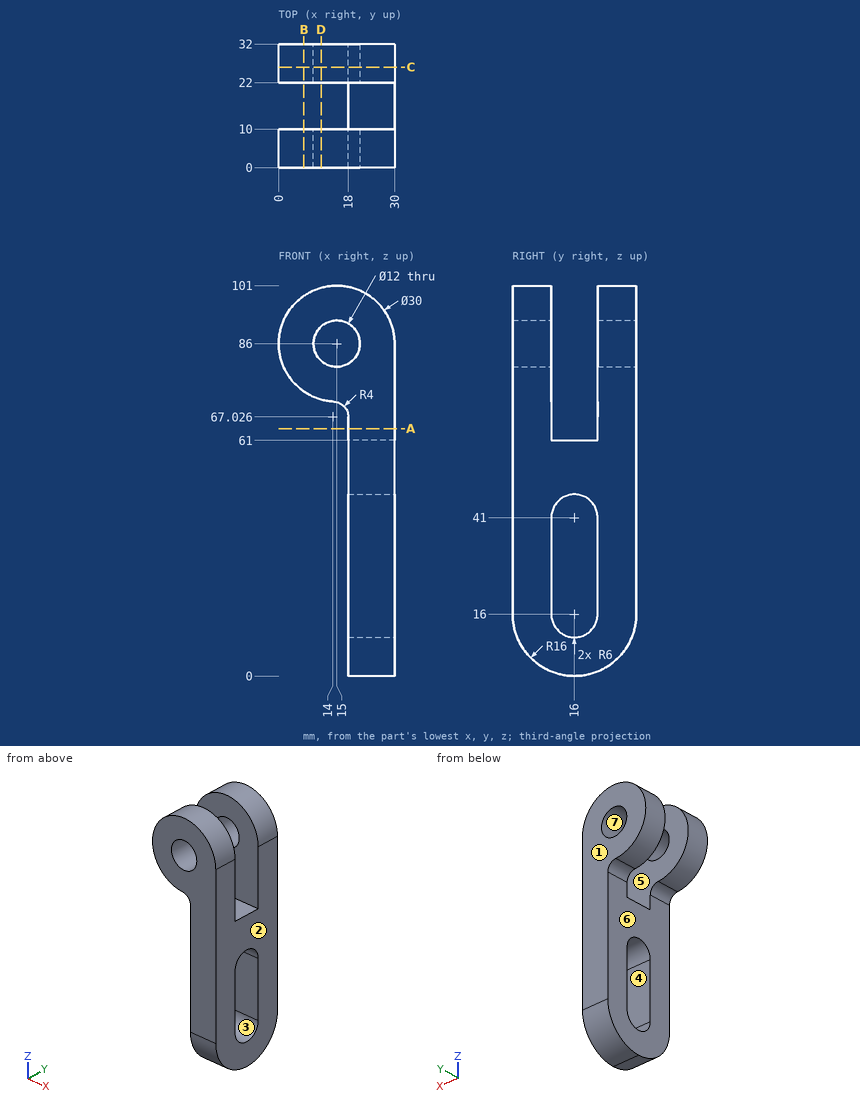
For this review, use the dimensioned drawing (mm, ordinates from the lowest corner) and the shaded views. A direction names the side the tool comes from. Round coordinates to 2 decimals unless told otherwise and drop trailing zeros. Write each loop counter-clockwise with the first axis right and the second up, starting at its lowest first coordinate (ties: lowest second). Pieces come first, ordered by that corner, then holes. Notation, with made-up numbers: (57.25, 70.25) -> (105.25, 70.25) arc R29 ccw to (105.25, 109.25) -> close; hole circle Ø11 at (51, 4). An arc over 180 degrees is marked (long way). Use CSV: the item, a comma, the result in double quotes.
Q1. Consider section A-A (z = 64). Give the boundary of the cut face in (x, y).
Checks:
outline,"(18, 0) -> (30, 0) -> (30, 10) -> (18, 10) -> close; (18, 22) -> (30, 22) -> (30, 32) -> (18, 32) -> close"
Q2. Consider section D-D (x = 11). Give the boundary of the cut face in (y, z), then the cut area to 3 significant figures.
Checks:
outline,"(0, 71.54) -> (10, 71.54) -> (10, 81.53) -> (0, 81.53) -> close; (0, 90.47) -> (10, 90.47) -> (10, 100.46) -> (0, 100.46) -> close; (22, 71.54) -> (32, 71.54) -> (32, 81.53) -> (22, 81.53) -> close; (22, 90.47) -> (32, 90.47) -> (32, 100.46) -> (22, 100.46) -> close"
area,"399 mm²"
Q3. Consider section B-B (x = 6.5). Give the boundary of the cut face in (y, z).
Checks:
outline,"(0, 73.64) -> (10, 73.64) -> (10, 98.36) -> (0, 98.36) -> close; (22, 73.64) -> (32, 73.64) -> (32, 98.36) -> (22, 98.36) -> close"
Q4. Consider section C-C (y = 26). Give the boundary of the cut face in (x, z), then the cut area to 3 significant figures.
Checks:
outline,"(14.21, 71.02) arc R4 cw to (18, 67.03) -> (18, 3.51) -> (30, 3.51) -> (30, 86) arc R15 ccw (long way) to start; hole circle Ø12 at (15, 86)"
area,"1,460 mm²"
Q5. For pin 1 Ø1 at (y, z) = (28, 91) entering from +X; pin 2 Ø9.5 at (x, y) = (27, 17) entering from +Z; pin 3 Ø9.5 at (y, z) = (8.5, 18.5) entering from -X, all flat-tipped, find the tip position at first contact; note any pin that passes through.
Checks:
pin 1,"x = 29.31"
pin 2,"z = 61"
pin 3,"x = 18"
Q6. For the marked faces 4, 5, 6 and 7, list the 3-axis set-ups (+Z, -Z, +X, -X, +Y, -Y) from which the entire face can be reached by the end or side of a thin tool; tool diameter is ignored.
Checks:
face 4,"+X, -X"
face 5,"+Z, +X, -X"
face 6,"-Z, -X, +Y, -Y"
face 7,"+Y, -Y"
Q7. To check wall thickness, follow probe 1 along Y at (x, z) = (8.5, 89.5); probe 2 along X at (y, z) = (6.5, 86); probe 3 along X at (y, z) = (23, 31.5). State the ranges of each line that lie inside material, in increasing order. Write a range as [from, to].
Checks:
probe 1,"[0, 10], [22, 32]"
probe 2,"[0, 9], [21, 30]"
probe 3,"[18, 30]"
Q8. Mouldability with a two-part tool opening along Y and no side actions: class the marked faces 1, 2 and 3 as released by +Y, released by -Y, zero draft, split by the parting line, or undercut.
Checks:
face 1,"released by +Y"
face 2,"zero draft"
face 3,"undercut"
